from build123d import *

# Parameters (mm, degrees)
F0_R     = 70
F0_R_2   = 60
F1_DEPTH = 3.5
F2_R     = 70
F2_R_2   = 56.5
F3_DEPTH = 5
F4_R     = 70
F4_R_2   = 56.5
F5_DEPTH = 5
F6_R     = 70
F7_DEPTH = 5


with BuildPart() as f1:
    # F0 (on Top) → F1 (new body)
    with BuildSketch(Plane.XY):
        Circle(F0_R)
        Circle(F0_R_2, mode=Mode.SUBTRACT)
    extrude(amount=F1_DEPTH)



with BuildPart() as f3:
    # F2 (on face) → F3 (new body)
    with BuildSketch(Plane(origin=(0, 0, -5), x_dir=(1, 0, 0), z_dir=(0, 0, -1))):
        Circle(F2_R)
        Circle(F2_R_2, mode=Mode.SUBTRACT)
    extrude(amount=F3_DEPTH)


with BuildPart() as f1_1:
    add(f1.part)

    add(f3.part)  # F5 merges F3
    # F4 (on face) → F5 (join)
    with BuildSketch(Plane(origin=(0, 0, 0), x_dir=(1, 0, 0), z_dir=(0, 0, -1))):
        Circle(F4_R)
        Circle(F4_R_2, mode=Mode.SUBTRACT)
    extrude(amount=F5_DEPTH)

    # F6 (on face) → F7 (join)
    with BuildSketch(Plane(origin=(0, 0, -10), x_dir=(1, 0, 0), z_dir=(0, 0, -1))):
        Circle(F6_R)
        with BuildLine():
            ThreePointArc((-32.822363, -21.05), (-36.459669, -21.05), (-34.641016, -17.9))
            ThreePointArc((-34.641016, -17.9), (-33.156092, -18.515076), (-32.541016, -20))
            ThreePointArc((-32.541016, -20), (-32.612572, -20.54352), (-32.822363, -21.05))
        make_face(mode=Mode.SUBTRACT)
        with BuildLine():
            ThreePointArc((2.1, -40), (-0.54352, -42.028444), (-1.818653, -38.95))
            ThreePointArc((-1.818653, -38.95), (0, -37.9), (1.818653, -38.95))
            ThreePointArc((1.818653, -38.95), (2.028444, -39.45648), (2.1, -40))
        make_face(mode=Mode.SUBTRACT)
        with BuildLine():
            ThreePointArc((36.741016, -20), (35.184536, -22.028444), (32.822363, -21.05))
            ThreePointArc((32.822363, -21.05), (32.822363, -18.95), (34.641016, -17.9))
            ThreePointArc((34.641016, -17.9), (36.12594, -18.515076), (36.741016, -20))
        make_face(mode=Mode.SUBTRACT)
        with BuildLine():
            ThreePointArc((-34.641016, 17.9), (-36.459669, 21.05), (-32.822363, 21.05))
            ThreePointArc((-32.822363, 21.05), (-32.612572, 20.54352), (-32.541016, 20))
            ThreePointArc((-32.541016, 20), (-33.156092, 18.515076), (-34.641016, 17.9))
        make_face(mode=Mode.SUBTRACT)
        with BuildLine():
            ThreePointArc((36.741016, 20), (36.12594, 18.515076), (34.641016, 17.9))
            ThreePointArc((34.641016, 17.9), (32.822363, 18.95), (32.822363, 21.05))
            ThreePointArc((32.822363, 21.05), (35.184536, 22.028444), (36.741016, 20))
        make_face(mode=Mode.SUBTRACT)
        with BuildLine():
            ThreePointArc((2.1, 40), (2.028444, 39.45648), (1.818653, 38.95))
            ThreePointArc((1.818653, 38.95), (0, 37.9), (-1.818653, 38.95))
            ThreePointArc((-1.818653, 38.95), (-0.54352, 42.028444), (2.1, 40))
        make_face(mode=Mode.SUBTRACT)
    extrude(amount=F7_DEPTH)


solid = f1_1.part
For this review, take the finished solid that the model builds, in its own axes (mm). A direction names the side the tool comes from. Give positions to 0.01 mm unless a question says otherwise; leave off trailing zeros. Order: outer loops, then holes, each group sorted by start corner. A loop starts at its lowest first (then second) coordinate and runs counter-clockwise, first axis right, second up. Notation, with made-up numbers: (-33, 3.5) - (6, 3.5) arc R33 cw to (6, 32.5) - close; hole circle Ø4 at (64.25, -20.5). An arc over 180 degrees is marked (long way). Answer as a JSON object with one key per item and string values. Group by question number.
Item 1: Clearance check with flat-ended pins moving along their axes: pin 1 Ø4 at (x, z) = (44.5, -7.5) entering from +Y; pin 2 Ø2 at (x, y) = (14.5, 54.5) entering from +Z; pin 3 Ø3 at (y, z) = (-46.5, -3) entering from +X; pin 4 Ø4 at (x, y) = (-34.64, -20) entering from +Z. State where each tip first meets the part, or that it passes through.
Item 2: Take a section at A-A on x = 0. Give the boundary of the cut face in (y, z), and give its area (3 significant figures).
Item 3: Machinability: for faces 4 (the flat face through (52, 31, 3.5)), 5 (the flat face through (22, 53, 0)), which of the approach directions +Z, -Z, +X, -X, +Y, -Y give a long, thin tool a straight path to every point of the face, cutting with its end or side? Answer none if there is none.
Item 4: Wall thickness on line 1 along X through (y, z) = (-20, -12.35); line 2 along Y through (x, z) = (0, 2.55); line 3 along Y through (x, z) = (0, -5.75): over which ranges is each line inside the solid? List them lowest first.
Item 5: Draft analysis for pull direction X (two halves, no side actions). For faces 1 (the flat face through (-1, -1, -15)), 2 (the cylindrical face through (-55.55, 42.594, -5.62)), 3 (the cylindrical face through (-59.94, 2.64, 1.73)), state which applies: pulls with the +X half, pulls with the -X half, needs draft (parallel to the pull), parting line crosses it, or undercut.
Item 6: Take a section at B-B on y = 33.5. Give the boundary of the cut face in (x, z), and give its area (3 significant figures).
Item 7: Take a section at D-D on x = -22.5. Give the boundary of the cut face in (y, z), and give its area (3 significant figures).
Item 8: Take a section at C-C on z = -3. Give the boundary of the cut face in (x, y).
Reported:
{
 "1": {"pin 1": "y = 55.62", "pin 2": "z = 0", "pin 3": "x = 53.62", "pin 4": "through"},
 "2": {"outline": "(-70, -15) - (-42.1, -15) - (-42.1, -10) - (-56.5, -10) - (-56.5, 0) - (-60, 0) - (-60, 3.5) - (-70, 3.5) - close; (-37.9, -15) - (37.9, -15) - (37.9, -10) - (-37.9, -10) - close; (42.1, -15) - (70, -15) - (70, 3.5) - (60, 3.5) - (60, 0) - (56.5, 0) - (56.5, -10) - (42.1, -10) - close", "area": "998 mm^2"},
 "3": {"face 4": "+Z, +X, -X, +Y, -Y", "face 5": "+Z"},
 "4": {"line 1": "-67.08 to -36.74, -32.54 to 32.54, 36.74 to 67.08", "line 2": "-70 to -60, 60 to 70", "line 3": "-70 to -56.5, 56.5 to 70"},
 "5": {"face 1": "needs draft", "face 2": "parting line crosses it", "face 3": "undercut"},
 "6": {"outline": "(-61.46, -15) - (61.46, -15) - (61.46, 3.5) - (49.78, 3.5) - (49.78, 0) - (45.5, 0) - (45.5, -10) - (-45.5, -10) - (-45.5, 0) - (-49.78, 0) - (-49.78, 3.5) - (-61.46, 3.5) - close", "area": "1,020 mm^2"},
 "7": {"outline": "(-66.29, -15) - (66.29, -15) - (66.29, 3.5) - (55.62, 3.5) - (55.62, 0) - (51.83, 0) - (51.83, -10) - (-51.83, -10) - (-51.83, 0) - (-55.62, 0) - (-55.62, 3.5) - (-66.29, 3.5) - close", "area": "1,030 mm^2"},
 "8": {"outline": "circle Ø140 at (0, 0); hole circle Ø113 at (0, 0)"}
}
